The listing builds one solid part. Answer for the finished solid, in the listing's coordinates (mm). A direction names the side the tool comes from. Round coordinates to 2 decimals unless told otherwise and drop trailing zeros. Write each loop counter-clockwise with the first axis right and the second up, starting at its lowest first coordinate (ties: lowest second). Pieces come first, ordered by that corner, then holes. Notation, with made-up numbers: (87.25, 68) - (115.25, 68) arc R9 ccw to (115.25, 74) - close; hole circle Ø10 at (-30.75, -2). An arc over 180 degrees is marked (long way). Answer as CSV lines item,"result". Start each with the question number.
Item 1: Which of the six approach directions +Z, -Z, +X, -X, +Y, -Y give full straight-line access (tool end or side, diameter ignored) to faces 1 (the flat face through (0, 15.875, 0)), 2 (the flat face through (-6.35, 8, 20)), 3 (the flat face through (-20, 8, 6.35))?
Item 2: A cutting plane is placed at D-D on z = 12.5. Determine the outline of the cut face in (x, y) (3 decimals).
Item 3: A cutting plane is placed at B-B on y = 13.5. State how many separate pieces and enclosed holes the cut face has, and give its area (3 significant figures).
Item 4: Straight lines are drawn through the part: line 1 along Z through (x, y) = (19, 2.5); line 2 along Z through (x, y) = (-15.5, 9); line 3 along Z through (x, y) = (19, 16.75). For each, find the intervals that lie inside material, in ascending order. Write a range as [from, to].
Item 5: For a pull along X with two mould halves and no side action, classify faces 4 (the cylindrical face through (11.28, 7.83, 11.17)), 5 (the flat face through (0, 18, 25.4)), 6 (the flat face through (25.4, 18, 0)) as pulls with the +X half, pulls with the -X half, needs draft (parallel to the pull), parting line crosses it, or undercut.
Item 6: A cutting plane is placed at C-C on x = 15.5. Determine the outline of the cut face in (y, z) (3 decimals), and give its area (3 significant figures).
Item 7: Flat-ended cylindrical pins translate along their axes: pin 1 (12 mm diameter, centred on x = 7, z = -0.5, fed in from -Y) (3 decimals); pin 2 (6 mm diameter, centred on x = 20.64, z = -20.64, fed in from -Y). Find the tip coordinate at first contact, or state that the pin passes through.
Item 8: A cutting plane is placed at A-A on x = -18.5. Determine the outline of the cut face in (y, z) (3 decimals).
```python
from build123d import *

# Parameters (mm, degrees)
SKETCH1_W               = 50.8
SKETCH1_H               = 50.8
BOSS_EXTRUDE1_DEPTH     = 19.05
F_1_4_CLEARANCE_HOLE1_D = 6.7564
SKETCH9_W               = 12.7
SKETCH9_H               = 12.7
CUT_EXTRUDE1_DEPTH      = 15.875


with BuildPart() as part:
    # Sketch1 → Boss-Extrude1 (new body)
    with BuildSketch(Plane(origin=(0, 0, 0), x_dir=(1, 0, 0), z_dir=(0, 1, 0))):
        Rectangle(SKETCH1_W, SKETCH1_H)
    extrude(amount=BOSS_EXTRUDE1_DEPTH)

    # 1/4 Clearance Hole1 (through all)
    with Locations(Plane(origin=(0, 19.05, 0), x_dir=(1, 0, 0), z_dir=(0, 1, 0))):
        with Locations((-20.6375, 20.6375), (20.6375, 20.6375), (20.6375, -20.6375), (-20.6375, -20.6375)):
            Hole(F_1_4_CLEARANCE_HOLE1_D / 2)

    # Sketch9 → Cut-Extrude1 (cut)
    with BuildSketch(Plane.XZ):
        with BuildLine():
            ThreePointArc((-6.35, 14.549677831), (-11.225320151, 11.225320151), (-14.549677831, 6.35))
            Line((-14.549677831, 6.35), (-6.35, 6.35))
            Line((-6.35, 6.35), (-6.35, 14.549677831))
        make_face()
        with BuildLine():
            Line((-6.35, 25.4), (-6.35, 14.549677831))
            ThreePointArc((-6.35, 14.549677831), (0, 15.875), (6.35, 14.549677831))
            Line((6.35, 14.549677831), (6.35, 25.4))
            Line((6.35, 25.4), (-6.35, 25.4))
        make_face()
        with BuildLine():
            Line((6.35, 14.549677831), (6.35, 6.35))
            Line((6.35, 6.35), (14.549677831, 6.35))
            ThreePointArc((14.549677831, 6.35), (11.225320151, 11.225320151), (6.35, 14.549677831))
        make_face()
        with BuildLine():
            Line((25.4, 6.35), (14.549677831, 6.35))
            ThreePointArc((14.549677831, 6.35), (15.540137718, 3.243415594), (15.875, 0))
            ThreePointArc((15.875, 0), (15.540137718, -3.243415594), (14.549677831, -6.35))
            Line((14.549677831, -6.35), (25.4, -6.35))
            Line((25.4, -6.35), (25.4, 6.35))
        make_face()
        with BuildLine():
            Line((14.549677831, -6.35), (6.35, -6.35))
            Line((6.35, -6.35), (6.35, -14.549677831))
            ThreePointArc((6.35, -14.549677831), (11.225320151, -11.225320151), (14.549677831, -6.35))
        make_face()
        with BuildLine():
            ThreePointArc((6.35, -14.549677831), (0, -15.875), (-6.35, -14.549677831))
            Line((-6.35, -14.549677831), (-6.35, -25.4))
            Line((-6.35, -25.4), (6.35, -25.4))
            Line((6.35, -25.4), (6.35, -14.549677831))
        make_face()
        with BuildLine():
            Line((-6.35, -6.35), (-14.549677831, -6.35))
            ThreePointArc((-14.549677831, -6.35), (-11.225320151, -11.225320151), (-6.35, -14.549677831))
            Line((-6.35, -14.549677831), (-6.35, -6.35))
        make_face()
        with BuildLine():
            Line((-14.549677831, 6.35), (-25.4, 6.35))
            Line((-25.4, 6.35), (-25.4, -6.35))
            Line((-25.4, -6.35), (-14.549677831, -6.35))
            ThreePointArc((-14.549677831, -6.35), (-15.875, 0), (-14.549677831, 6.35))
        make_face()
        with BuildLine():
            Line((-6.35, 6.35), (-14.549677831, 6.35))
            ThreePointArc((-14.549677831, 6.35), (-15.875, 0), (-14.549677831, -6.35))
            Line((-14.549677831, -6.35), (-6.35, -6.35))
            Line((-6.35, -6.35), (-6.35, 6.35))
        make_face()
        with BuildLine():
            Line((6.35, -6.35), (-6.35, -6.35))
            Line((-6.35, -6.35), (-6.35, -14.549677831))
            ThreePointArc((-6.35, -14.549677831), (0, -15.875), (6.35, -14.549677831))
            Line((6.35, -14.549677831), (6.35, -6.35))
        make_face()
        with BuildLine():
            Line((14.549677831, 6.35), (6.35, 6.35))
            Line((6.35, 6.35), (6.35, -6.35))
            Line((6.35, -6.35), (14.549677831, -6.35))
            ThreePointArc((14.549677831, -6.35), (15.540137718, -3.243415594), (15.875, 0))
            ThreePointArc((15.875, 0), (15.540137718, 3.243415594), (14.549677831, 6.35))
        make_face()
        Rectangle(SKETCH9_W, SKETCH9_H)
        with BuildLine():
            Line((-6.35, 14.549677831), (-6.35, 6.35))
            Line((-6.35, 6.35), (6.35, 6.35))
            Line((6.35, 6.35), (6.35, 14.549677831))
            ThreePointArc((6.35, 14.549677831), (0, 15.875), (-6.35, 14.549677831))
        make_face()
    extrude(amount=-CUT_EXTRUDE1_DEPTH, mode=Mode.SUBTRACT)


solid = part.part
```
Geometry says:
1,face 1,"-Y"
1,face 2,"+Z, -Z, -Y"
1,face 3,"+X, -X, -Y"
2,outline,"(-25.4, 0) - (-9.786, 0) - (-9.786, 15.875) - (9.786, 15.875) - (9.786, 0) - (25.4, 0) - (25.4, 19.05) - (-25.4, 19.05) - close"
3,separate pieces,"4"
3,enclosed holes,"4"
3,area,"1,140 mm^2"
4,line 1,"z = [-25.4, -23.59], [-17.68, -6.35], [6.35, 17.68], [23.59, 25.4]"
4,line 2,"z = [-25.4, -6.35], [6.35, 25.4]"
4,line 3,"z = [-25.4, -23.59], [-17.68, 17.68], [23.59, 25.4]"
5,face 4,"undercut"
5,face 5,"needs draft"
5,face 6,"pulls with the +X half"
6,outline,"(0, -25.4) - (19.05, -25.4) - (19.05, 25.4) - (0, 25.4) - (0, 6.35) - (15.875, 6.35) - (15.875, -6.35) - (0, -6.35) - close"
6,area,"766 mm^2"
7,pin 1,"stops at y = 15.875"
7,pin 2,"passes through"
8,outline,"(0, -25.4) - (19.05, -25.4) - (19.05, -23.253) - (0, -23.253) - close; (0, -18.022) - (19.05, -18.022) - (19.05, 18.022) - (0, 18.022) - (0, 6.35) - (15.875, 6.35) - (15.875, -6.35) - (0, -6.35) - close; (0, 23.253) - (19.05, 23.253) - (19.05, 25.4) - (0, 25.4) - close"
